CAD build for the part. Positions are in the model's coordinates, mm. A direction names the side the tool comes from. Give positions to 0.01 mm unless a question says otherwise; leave off trailing zeros. Order: outer loops, then holes, each group sorted by start corner. A loop starts at its lowest first (then second) coordinate and runs counter-clockwise, first axis right, second up. Notation, with made-up numbers: (68.5, -7.5) -> (105.5, -7.5) arc R21 cw to (105.5, 17.5) -> close; hole circle Ø6 at (78.25, -12.5). An arc over 180 degrees is marked (long way). Use one line per item in the form item = value. Start each with the question number.
1) Probe line 1 (Y direction, x = 16, z = -5.8); line 2 (Y direction, x = 69, z = -1.55); line 3 (Z direction, x = 18.5, y = 14). List the from-to ranges inside material, lowest first.
2) Mould opens along Z. For faces 1 (the face through (-7.5, -8.65, 0.16)), 2 (the face through (36.414, 0.224, -2.642)), 3 (the face through (19, 11, 5)) say: pulls with the +Z half, pulls with the -Z half, needs draft (parallel to the pull), parting line crosses it, or undercut.
3) Drop flat-ended pins along their axis: P1, Ø2, axis at y = -6, z = -2.5, coming from the +X side; P2, Ø10, axis at x = 68, y = 3.5, coming from the -Z side; P3, Ø3, axis at y = -1, z = -3.5, coming from the +X side; P4, Ø5, axis at x = 83, y = 6.5, coming from the +Z side. Give the stop position or say it passes through.
4) Cut at B-B, the plane x = 16. Give the cut face in (y, z).
5) Cut at D-D, the plane y = -7.5. Give the cut face in (x, z).
6) Cut at A-A, the plane x = 79. Give the cut face in (y, z).
7) Cut at C-C, the plane z = 2.5. Give the cut face in (x, y), and give its area (3 significant figures).
8) Tool access for faces 4 (the face through (32.31, 0.22, -4.86)), 5 (the face through (-5.3, 1.5, -0.1)), 6 (the face through (93.851, 15.274, -1.232)), 7 (the face through (31.1, -15.14, 6.27)): list every direction of +Z, -Z, +X, -X, +Y, -Y with a clear straight run to the whole face (end or side of a thin tool).
from build123d import *

# Parameters (mm, degrees)
BASE_FLANGE1_DEPTH      = 16
CUT_EXTRUDE1_START      = -15
CUT_EXTRUDE1_DEPTH      = 15
SKETCH7_R               = 3.25
CUT_EXTRUDE2_DEPTH      = 10
CUT_EXTRUDE3_DEPTH      = 98.612755314
CUT_EXTRUDE3_DEPTH_BACK = 2.5
FILLET1_R               = 3


# Read off the part's stored shape, not the designer's step: Cut-Extrude1
# Sheet-metal steps are written as plain solids
with BuildPart() as part:
    # Sketch1 → Base-Flange1 (new, symmetric)
    with BuildSketch(Plane(origin=(0, 0, 0), x_dir=(1, 0, 0), z_dir=(0, 1, 0))):
        with BuildLine():
            Line((32, -7.5), (0, -7.5))
            ThreePointArc((0, -7.5), (-7.5, 0), (0, 7.5))
            Line((0, 7.5), (31.258330249, 7.5))
            ThreePointArc((31.258330249, 7.5), (32.940654042, 7.278517871), (34.508330249, 6.629165125))
            Line((34.508330249, 6.629165125), (40.732050808, 3.035898385))
            ThreePointArc((40.732050808, 3.035898385), (41.696774627, 2.636296695), (42.732050808, 2.5))
            Line((42.732050808, 2.5), (96, 2.5))
            Line((96, 2.5), (96, 0))
            Line((96, 0), (42.732050808, 0))
            ThreePointArc((42.732050808, 0), (41.049727014, 0.221482129), (39.482050808, 0.870834875))
            Line((39.482050808, 0.870834875), (33.258330249, 4.464101615))
            ThreePointArc((33.258330249, 4.464101615), (32.29360643, 4.863703305), (31.258330249, 5))
            Line((31.258330249, 5), (0, 5))
            ThreePointArc((0, 5), (-5, 0), (0, -5))
            Line((0, -5), (32, -5))
            Line((32, -5), (32, -7.5))
        make_face()
    extrude(amount=BASE_FLANGE1_DEPTH, both=True)

    # Cut-Extrude1 outline → Cut-Extrude1 (cut)
    with BuildSketch(Plane.XY.offset(7.5).offset(CUT_EXTRUDE1_START)):
        with BuildLine():
            Line((5.102752641, 1.5), (-7.5, 1.5))
            Line((-7.5, 1.5), (-7.5, -1.5))
            Line((-7.5, -1.5), (5.102752641, -1.5))
            ThreePointArc((5.102752641, -1.5), (27, 0), (5.102752641, 1.5))
        make_face()
    extrude(amount=CUT_EXTRUDE1_DEPTH, mode=Mode.SUBTRACT)

    # Sketch7 → Cut-Extrude2 (cut)
    with BuildSketch(Plane.XY):
        with Locations((79, 0)):
            Circle(SKETCH7_R)
        with Locations((69, 0)):
            Circle(SKETCH7_R)
    extrude(amount=-CUT_EXTRUDE2_DEPTH, mode=Mode.SUBTRACT)

    # Sketch8 → Cut-Extrude3 (cut, two sides: drawn at the far end of the back side and taken through both)
    with BuildSketch(Plane.XY.offset(-CUT_EXTRUDE3_DEPTH_BACK)):
        with BuildLine():
            Line((49.66733752, 235.064404157), (94.383671769, 16))
            ThreePointArc((94.383671769, 16), (96, 0), (94.383671769, -16))
            Line((94.383671769, -16), (49.66733752, -235.064404157))
            Line((49.66733752, -235.064404157), (496.830680013, -235.064404157))
            Line((496.830680013, -235.064404157), (496.830680013, 235.064404157))
            Line((496.830680013, 235.064404157), (49.66733752, 235.064404157))
        make_face()
    extrude(amount=CUT_EXTRUDE3_DEPTH + CUT_EXTRUDE3_DEPTH_BACK, mode=Mode.SUBTRACT)

    # Fillet1
    fillet1_edges = [part.edges().sort_by_distance(p)[0] for p in [
        (94.383671769, 16, -1.25),
        (94.383671769, -16, -1.25),
        (32, -16, 6.25),
        (32, 16, 6.25),
    ]]
    fillet(fillet1_edges, radius=FILLET1_R)


solid = part.part
Result:
q1.line_1 = -16 to -11, 11 to 16
q1.line_2 = -16 to -3.25, 3.25 to 16
q1.line_3 = -7.5 to -5, 5 to 7.5
q2.face_1 = parting line crosses it
q2.face_2 = pulls with the +Z half
q2.face_3 = undercut
q3.P1 = 95.84
q3.P2 = -2.5
q3.P3 = 96
q3.P4 = 0
q4.outline = (-16, -7.5) -> (-11, -7.5) -> (-11, -5) -> (-16, -5) -> close; (-16, 5) -> (-11, 5) -> (-11, 7.5) -> (-16, 7.5) -> close; (11, -7.5) -> (16, -7.5) -> (16, -5) -> (11, -5) -> close; (11, 5) -> (16, 5) -> (16, 7.5) -> (11, 7.5) -> close
q5.outline = (0, -7.5) -> (7.95, -7.5) -> (7.95, -5) -> (0, -5) arc R5 cw to (0, 5) -> (7.95, 5) -> (7.95, 7.5) -> (0, 7.5) arc R7.5 ccw to start; (24.05, -7.5) -> (31.26, -7.5) arc R6.5 ccw to (34.51, -6.63) -> (40.73, -3.04) arc R4 cw to (42.73, -2.5) -> (95.65, -2.5) -> (95.65, 0) -> (42.73, 0) arc R6.5 ccw to (39.48, -0.87) -> (33.26, -4.46) arc R4 cw to (31.26, -5) -> (24.05, -5) -> close; (24.05, 5) -> (32, 5) -> (32, 7.5) -> (24.05, 7.5) -> close
q6.outline = (-16, -2.5) -> (-3.25, -2.5) -> (-3.25, 0) -> (-16, 0) -> close; (3.25, -2.5) -> (16, -2.5) -> (16, 0) -> (3.25, 0) -> close
q7.outline = (-7.07, -16) -> (-4.33, -16) -> (-4.33, -1.5) -> (-7.07, -1.5) -> close; (-7.07, 1.5) -> (-4.33, 1.5) -> (-4.33, 16) -> (-7.07, 16) -> close
q7.area = 79.5 mm²
q8.face_4 = +Y, -Y
q8.face_5 = +Z, -Z, -X
q8.face_6 = +Z, -Z, +X, +Y
q8.face_7 = +Z, +X, -Y
